Geometry check sheet. Reference: the model listing, model coordinates, mm. A direction names the side the tool comes from. Coordinates: 2 decimals unless noted, no trailing zeros. Order: outer loops, then holes, each group sorted by start corner. A loop starts at its lowest first (then second) coordinate and runs counter-clockwise, first axis right, second up. Notation, with made-up numbers: (-19, -2) - (-8, -2) arc R16 cw to (-8, 11) - close; hole circle Ø5 at (-5, -6). An arc over 180 degrees is marked (long way). Put each result on its own line as item: value.
from build123d import *

# Parameters (mm, degrees)
F0_W          = 40.386
F0_H          = 20.32
F1_DEPTH      = 27.432
F1_DEPTH_BACK = 11.684
F2_R          = 1.905
F3_DEPTH      = 2.54
F4_R          = 2.921
F5_DEPTH      = 5.334


with BuildPart() as f1:
    # F0 (on Top) → F1 (new body, two sides)
    with BuildSketch(Plane.XY) as f1_sk:
        Rectangle(F0_W, F0_H)
    extrude(amount=-F1_DEPTH)
    extrude(f1_sk.sketch, amount=F1_DEPTH_BACK)

    # F2 (on Top) → F3 (join)
    with BuildSketch(Plane.XY):
        with BuildLine():
            Line((26.035, 10.16), (-26.035, 10.16))
            ThreePointArc((-26.035, 10.16), (-27.4718409794, 9.5648409794), (-28.067, 8.128))
            Line((-28.067, 8.128), (-28.067, -8.128))
            ThreePointArc((-28.067, -8.128), (-27.4718409794, -9.5648409794), (-26.035, -10.16))
            Line((-26.035, -10.16), (26.035, -10.16))
            ThreePointArc((26.035, -10.16), (27.4718409794, -9.5648409794), (28.067, -8.128))
            Line((28.067, -8.128), (28.067, 8.128))
            ThreePointArc((28.067, 8.128), (27.4718409794, 9.5648409794), (26.035, 10.16))
        make_face()
        with Locations((-23.495, -4.445)):
            Circle(F2_R, mode=Mode.SUBTRACT)
        with Locations((23.495, -4.445)):
            Circle(F2_R, mode=Mode.SUBTRACT)
        with Locations((-23.495, 4.445)):
            Circle(F2_R, mode=Mode.SUBTRACT)
        with Locations((23.495, 4.445)):
            Circle(F2_R, mode=Mode.SUBTRACT)
    extrude(amount=F3_DEPTH)

    # F4 (on face) → F5 (join)
    with BuildSketch(Plane.XY.offset(11.684)):
        with Locations((-10.16, 0)):
            Circle(F4_R)
    extrude(amount=F5_DEPTH)


solid = f1.part
Q1. Section check C-C on z = -21.5. Record the boundary of the cut face in (x, y).
Answer block:
outline: (-20.19, -10.16) - (20.19, -10.16) - (20.19, 10.16) - (-20.19, 10.16) - close
Q2. Thickness scan on L1, parallel to X at y = -2, z = -20; L2, parallel to Z at x = 19.5, y = 4; L3, parallel to X at y = 0.25, z = 13. Record the ranges inside material, lowest first. Write a range as [from, to].
Answer block:
L1: x = [-20.19, 20.19]
L2: z = [-27.43, 11.68]
L3: x = [-13.07, -7.25]
Q3. Access from +Z, -Z, +X, -X, +Y, -Y to the whole of each face (thin tool, end or side, straight path). Record for faces 1 (the flat face through (24, 0, 0)), 2 (the flat face through (-20.193, 0, 7)), 3 (the flat face through (20.193, 0, 7)).
Answer block:
face 1: -Z, +X, +Y, -Y
face 2: +Z, -X, +Y, -Y
face 3: +Z, +X, +Y, -Y
Q4. Section check A-A on y = -7. Record the boundary of the cut face in (x, z).
Answer block:
outline: (-28.07, 0) - (-20.19, 0) - (-20.19, -27.43) - (20.19, -27.43) - (20.19, 0) - (28.07, 0) - (28.07, 2.54) - (20.19, 2.54) - (20.19, 11.68) - (-20.19, 11.68) - (-20.19, 2.54) - (-28.07, 2.54) - close
Q5. Depth check by flat-ended pin: pin 1 Ø7.5 at (y, z) = (-0.5, 6.5) entering from -X; pin 2 Ø6.5 at (x, y) = (25, 5) entering from +Z; pin 3 Ø8.5 at (x, y) = (25, 5) entering from -Z. Enter the tip coordinate at first touch or a pass-through.
Answer block:
pin 1: stops at x = -20.19
pin 2: stops at z = 2.54
pin 3: stops at z = 0
Q6. Section check D-D on y = 0. Record the boundary of the cut face in (x, z), then the cut area to 3 significant figures.
Answer block:
outline: (-28.07, 0) - (-20.19, 0) - (-20.19, -27.43) - (20.19, -27.43) - (20.19, 0) - (28.07, 0) - (28.07, 2.54) - (20.19, 2.54) - (20.19, 11.68) - (-7.24, 11.68) - (-7.24, 17.02) - (-13.08, 17.02) - (-13.08, 11.68) - (-20.19, 11.68) - (-20.19, 2.54) - (-28.07, 2.54) - close
area: 1,650 mm^2
Q7. Draft check along Y on faces 4 (the cylindrical face through (21.59, 4.53, 1.25)), 5 (the cylindrical face through (-25.4, 4.5, 1.3)), 6 (the cylindrical face through (-27.456, 9.581, 1.252)), 7 (the flat face through (0, 0, -27.432)). Enter one of: pulls with the +Y half, pulls with the -Y half, needs draft (parallel to the pull), parting line crosses it, or undercut.
Answer block:
face 4: undercut
face 5: undercut
face 6: pulls with the +Y half
face 7: needs draft
Q8. Section check B-B on x = -10.16. Record the boundary of the cut face in (y, z), then the cut area to 3 significant figures.
Answer block:
outline: (-10.16, -27.43) - (10.16, -27.43) - (10.16, 11.68) - (2.92, 11.68) - (2.92, 17.02) - (-2.92, 17.02) - (-2.92, 11.68) - (-10.16, 11.68) - close
area: 826 mm^2
